from build123d import *

# Parameters (mm, degrees)
BOSS_EXTRU_1_DEPTH      = 20
ESQUISSE3_R             = 1.5
ENL_V_MAT_EXTRU_3_DEPTH = 20
ESQUISSE4_R             = 1.5
ENL_V_MAT_EXTRU_4_DEPTH = 10
ESQUISSE5_R             = 1.5
ENL_V_MAT_EXTRU_5_DEPTH = 10


with BuildPart() as part:
    # Esquisse1 → Boss.-Extru.1 (new body)
    with BuildSketch(Plane(origin=(0, 0, 0), x_dir=(1, 0, 0), z_dir=(0, 1, 0))):
        with BuildLine():
            Line((-3, 84.398281038), (-3, 69.398281038))
            Line((-3, 69.398281038), (-7, 69.398281038))
            Line((-7, 69.398281038), (-7, 65.398281038))
            Line((-7, 65.398281038), (-3, 65.398281038))
            Line((-3, 65.398281038), (-3, 54.398281038))
            Line((-3, 54.398281038), (-18.71, 54.398281038))
            ThreePointArc((-18.71, 54.398281038), (-22.308577777, 49.499317693), (-26.183329952, 44.81574006))
            ThreePointArc((-26.183329952, 44.81574006), (-12.83252844, 48.159570073), (-5, 36.842476876))
            Line((-5, 36.842476876), (-5, -39.182739587))
            Line((-5, -39.182739587), (0, -39.182739587))
            Line((0, -39.182739587), (0, 84.398281038))
            Line((0, 84.398281038), (-3, 84.398281038))
        make_face()
    boss_extru_1 = extrude(amount=BOSS_EXTRU_1_DEPTH)

    # Symétrie1: Boss.-Extru.1 across plane
    add(boss_extru_1.mirror(Plane(origin=(0, 20, -84.398281038), x_dir=(0, 0, 1), z_dir=(-1, 0, 0))))

    # Esquisse3 → Enlèv. mat.-Extru.3 (cut)
    with BuildSketch(Plane.ZY.offset(3)):
        with Locations((-76.398281038, 10)):
            Circle(ESQUISSE3_R)
        with Locations((-60.398281038, 10)):
            Circle(ESQUISSE3_R)
    extrude(amount=-ENL_V_MAT_EXTRU_3_DEPTH, mode=Mode.SUBTRACT)

    # Esquisse4 → Enlèv. mat.-Extru.4 (cut)
    with BuildSketch(Plane.ZY.offset(5)):
        with Locations((29.291975875, 10.84)):
            Circle(ESQUISSE4_R)
    extrude(amount=-ENL_V_MAT_EXTRU_4_DEPTH, mode=Mode.SUBTRACT)

    # Esquisse5 → Enlèv. mat.-Extru.5 (cut)
    with BuildSketch(Plane.ZY.offset(5)):
        with Locations((17.841975875, 10.84)):
            Circle(ESQUISSE5_R)
    extrude(amount=-ENL_V_MAT_EXTRU_5_DEPTH, mode=Mode.SUBTRACT)


solid = part.part
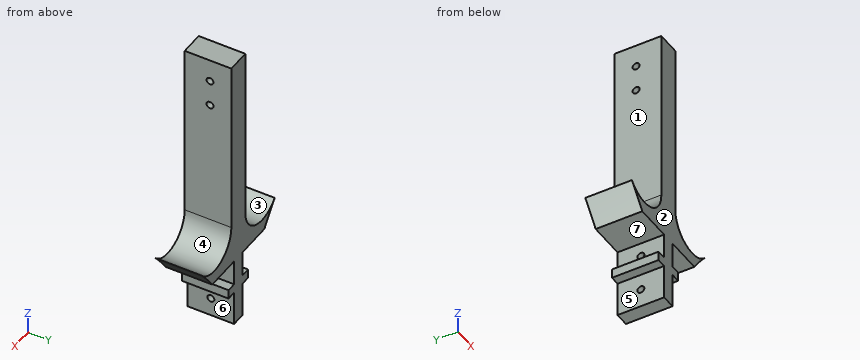
Could you check a few things on this model? Use its own coordinates, in mm. Face numbers are marked on the shaded views. A direction names the side the tool comes from. Give positions to 0.01 mm unless a question says otherwise; leave off trailing zeros. Order: outer loops, then holes, each group sorted by start corner. A loop starts at its lowest first (then second) coordinate and runs counter-clockwise, first axis right, second up. Notation, with made-up numbers: M 12.25,75.25 L 61.25,75.25 A31 cw 61.25,111.25 Z; hole C 17,68 d1. An arc over 180 degrees is marked long. One line per question, with ' | ' between items.
1. We'd pull the mould along X, two halves only. Please class the marked faces 1, 2, 3 and 4: +X half, -X half, draft (parallel to the pull), parting line (faces both ways), or undercut.
Results:
face 1: -X half | face 2: draft | face 3: undercut | face 4: undercut
2. For the marked faces 5, 6 and 7, which set-ups out of +Z, -Z, +X, -X, +Y, -Y let a thin tool reach every point of the face, with its end or its side?
Results:
face 5: -Z, -X, +Y, -Y | face 6: -Z, +X, +Y, -Y | face 7: -X, +Y, -Y
3. I want a section at C-C (x = -12.5). List the corners of the cut face in (y, z) for me.
Results:
outline: M 0,-54.4 L 20,-54.4 L 20,-48.03 L 0,-48.03 Z
4. If I drill on line 1 (Z direction, x = 2.5, y = 11.75); line 2 (X direction, y = 6.25, z = 0); line 3 (X direction, y = 1.25, z = -61.5), over which ranges is the centre line in solid material (lowest first)?
Results:
line 1: -84.4 to 16.65, 19.03 to 28.1, 30.48 to 39.18 | line 2: -5 to 5 | line 3: -3 to 3
5. I'm going to push flat-ended pins straight in: pin 1 (5.5 mm diameter, centred on y = 14.5, z = -58, fed in from -X); pin 2 (4.5 mm diameter, centred on x = 13.5, y = 9, fed in from -Z); pin 3 (7.5 mm diameter, centred on y = 10.5, z = -73, fed in from -X); pin 4 (2.5 mm diameter, centred on y = 10.84, z = 17.84, fed in from -X). Where does each tip first touch, or does it pass through?
Results:
pin 1: x = -3 | pin 2: z = -54.4 | pin 3: x = -7 | pin 4: through
6. I want a section at A-A (y = 3.5). List the corners of the cut face in (x, z) for me, and give its area (3 significant figures).
Results:
outline: M -26.18,-44.82 A105.5 cw -18.71,-54.4 L -3,-54.4 L -3,-65.4 L -7,-65.4 L -7,-69.4 L -3,-69.4 L -3,-84.4 L 3,-84.4 L 3,-69.4 L 7,-69.4 L 7,-65.4 L 3,-65.4 L 3,-54.4 L 18.71,-54.4 A105.5 cw 26.18,-44.82 A12.09 cw 5,-36.84 L 5,39.18 L -5,39.18 L -5,-36.84 A12.09 cw Z | area: 1,390 mm²
7. I want a section at B-B (z = -3). List the corners of the cut face in (x, y) for me.
Results:
outline: M -5,0 L 5,0 L 5,20 L -5,20 Z
